Input: part model. Units: mm. Frame: model coordinates. A direction names the side the tool comes from. Give positions to 0.01 mm unless a question says otherwise; leave off trailing zeros. Loops run counter-clockwise (first coordinate to the right, second up) from the corner with the lowest first, then second, coordinate; pieces in that order, holes last. Notation, with made-up numbers: (5.5, 39.25) - (9.5, 39.25) arc R30 ccw to (9.5, 72.25) - close; hole circle Ø4 at (68, 68.25). An arc over 180 degrees is marked (long way). Answer as a JSON object with one key per item and string values.
from build123d import *

# Parameters (mm, degrees)
SKETCH3_W           = 29.5
SKETCH3_H           = 13
BOSS_EXTRUDE2_DEPTH = 7.2
SKETCH5_R           = 1.6
BOSS_EXTRUDE3_DEPTH = 1.5
SKETCH9_W           = 8.95
SKETCH9_H           = 11.9
SKETCH9_W_2         = 10.45
BOSS_EXTRUDE4_DEPTH = 14.4
SKETCH10_W          = 10.1
SKETCH10_H          = 8.4
BOSS_EXTRUDE5_DEPTH = 9.9
SKETCH11_W          = 6.95
SKETCH11_H          = 9.9
SKETCH11_W_2        = 8.45
CUT_EXTRUDE2_DEPTH  = 5
FILLET2_R           = 1


with BuildPart() as part:
    # Sketch3 → Boss-Extrude2 (new body)
    with BuildSketch(Plane(origin=(0, 0, 0), x_dir=(1, 0, 0), z_dir=(0, 1, 0))):
        Rectangle(SKETCH3_W, SKETCH3_H)
    extrude(amount=BOSS_EXTRUDE2_DEPTH)

    # Sketch5 → Boss-Extrude3 (add)
    with BuildSketch(Plane(origin=(0, 0, 0), x_dir=(1, 0, 0), z_dir=(0, 1, 0))):
        with BuildLine():
            Line((-18.5, 3.75), (-14.75, 3.75))
            Line((-14.75, 3.75), (-14.75, -3.75))
            Line((-14.75, -3.75), (-18.5, -3.75))
            ThreePointArc((-18.5, -3.75), (-22.25, 0), (-18.5, 3.75))
        make_face()
        with Locations(Location((-18.5, 0, 0), (0, 0, 270))):
            Circle(SKETCH5_R, mode=Mode.SUBTRACT)
    boss_extrude3 = extrude(amount=BOSS_EXTRUDE3_DEPTH)

    # Mirror1: Boss-Extrude3 across plane
    add(boss_extrude3.mirror(Plane(origin=(0, 0, 0), x_dir=(0, 0, 1), z_dir=(1, 0, 0))))

    # Sketch9 → Boss-Extrude4 (add)
    with BuildSketch(Plane(origin=(0, 7.2, 0), x_dir=(1, 0, 0), z_dir=(0, 1, 0))):
        with Locations((-10.275, 0)):
            Rectangle(SKETCH9_W, SKETCH9_H)
        with Locations((9.525, 0)):
            Rectangle(SKETCH9_W_2, SKETCH9_H)
    extrude(amount=BOSS_EXTRUDE4_DEPTH)

    # Sketch10 → Boss-Extrude5 (add)
    with BuildSketch(Plane(origin=(0, 7.2, 0), x_dir=(1, 0, 0), z_dir=(0, 1, 0))):
        with Locations((-0.75, -0.057461808)):
            Rectangle(SKETCH10_W, SKETCH10_H)
    extrude(amount=BOSS_EXTRUDE5_DEPTH)

    # Sketch11 → Cut-Extrude2 (cut)
    with BuildSketch(Plane(origin=(0, 21.6, 0), x_dir=(1, 0, 0), z_dir=(0, 1, 0))):
        with Locations((-10.275, 0)):
            Rectangle(SKETCH11_W, SKETCH11_H)
        with Locations((9.525, 0)):
            Rectangle(SKETCH11_W_2, SKETCH11_H)
    extrude(amount=-CUT_EXTRUDE2_DEPTH, mode=Mode.SUBTRACT)

    # Fillet2
    fillet2_edges = [part.edges().sort_by_distance(p)[0] for p in [
        (-14.75, 14.4, -5.95),
        (-14.75, 14.4, 5.95),
        (-5.8, 14.4, 5.95),
        (-5.8, 14.4, -5.95),
        (14.75, 14.4, 5.95),
        (14.75, 14.4, -5.95),
        (4.3, 14.4, -5.95),
        (4.3, 14.4, 5.95),
        (-13.75, 19.1, 4.95),
        (-13.75, 19.1, -4.95),
        (-6.8, 19.1, -4.95),
        (-6.8, 19.1, 4.95),
        (5.3, 19.1, 4.95),
        (5.3, 19.1, -4.95),
        (13.75, 19.1, -4.95),
        (13.75, 19.1, 4.95),
    ]]
    fillet(fillet2_edges, radius=FILLET2_R)


solid = part.part
Item 1: Cut plane A-A (z = 0). Return loops of the section in (x, y), then the cut area to 3 significant figures.
Geometry check:
{"outline": "(-22.25, 0) - (-20.1, 0) - (-20.1, 1.5) - (-22.25, 1.5) - close; (-16.9, 0) - (16.9, 0) - (16.9, 1.5) - (14.75, 1.5) - (14.75, 21.6) - (13.75, 21.6) - (13.75, 16.6) - (5.3, 16.6) - (5.3, 21.6) - (4.3, 21.6) - (4.3, 17.1) - (-5.8, 17.1) - (-5.8, 21.6) - (-6.8, 21.6) - (-6.8, 16.6) - (-13.75, 16.6) - (-13.75, 21.6) - (-14.75, 21.6) - (-14.75, 1.5) - (-16.9, 1.5) - close; (20.1, 0) - (22.25, 0) - (22.25, 1.5) - (20.1, 1.5) - close", "area": "528 mm2"}
Item 2: Material intervals for line 1 (X direction, y = 0.5, z = 0); line 2 (X direction, y = 17.25, z = -0.5); line 3 (X direction, y = 19.25, z = -4.25), sorted ascending. Write a range as [from, to].
Geometry check:
{"line 1": "x = [-22.25, -20.1], [-16.9, 16.9], [20.1, 22.25]", "line 2": "x = [-14.75, -13.75], [-6.8, -5.8], [4.3, 5.3], [13.75, 14.75]", "line 3": "x = [-14.75, -13.7], [-6.85, -5.8], [4.3, 5.35], [13.7, 14.75]"}
Item 3: Mould query, pull axis X, two halves, no side actions, for faces 5 (the face through (5.601, 19.065, -4.665)), 6 (the face through (17, 1, 3.75)). Classes: released by +X, released by -X, zero draft, split by the parting line, or undercut.
Geometry check:
{"face 5": "undercut", "face 6": "zero draft"}
Item 4: Contact query for flat-ended pins moving along their axis: P1, Ø1.5, axis at x = 8.5, y = 18, coming from the -Z side; P2, Ø2, axis at x = 10.5, y = 15.5, coming from the +Z side; P3, Ø3.5, axis at x = -9.5, z = 1.5, coming from the +Y side. Output: stop coordinate, or through.
Geometry check:
{"P1": "stops at z = -5.95", "P2": "stops at z = 5.95", "P3": "stops at y = 16.6"}
Item 5: Cut plane B-B (x = -1). Return loops of the section in (y, z), then the cut area to 3 significant figures.
Geometry check:
{"outline": "(0, -6.5) - (7.2, -6.5) - (7.2, -4.14) - (17.1, -4.14) - (17.1, 4.26) - (7.2, 4.26) - (7.2, 6.5) - (0, 6.5) - close", "area": "177 mm2"}
Item 6: Cut plane C-C (y = 9.5). Return loops of the section in (x, z).
Geometry check:
{"outline": "(-14.75, -4.95) arc R1 ccw to (-13.75, -5.95) - (-6.8, -5.95) arc R1 ccw to (-5.8, -4.95) - (-5.8, -4.14) - (4.3, -4.14) - (4.3, -4.95) arc R1 ccw to (5.3, -5.95) - (13.75, -5.95) arc R1 ccw to (14.75, -4.95) - (14.75, 4.95) arc R1 ccw to (13.75, 5.95) - (5.3, 5.95) arc R1 ccw to (4.3, 4.95) - (4.3, 4.26) - (-5.8, 4.26) - (-5.8, 4.95) arc R1 ccw to (-6.8, 5.95) - (-13.75, 5.95) arc R1 ccw to (-14.75, 4.95) - close"}
Item 7: Cut plane D-D (y = 3.25). Return loops of the section in (x, z), then the cut area to 4 significant figures.
Geometry check:
{"outline": "(-14.75, -6.5) - (14.75, -6.5) - (14.75, 6.5) - (-14.75, 6.5) - close", "area": "383.5 mm2"}
Item 8: Access query for faces 1 (the face through (9, 14, 5.95)), 2 (the face through (0, 7.2, -6)), 3 (the face through (-7.085, 19.065, -4.649)), 4 (the face through (0, 7.2, 6)). Directions: +Z, -Z, +X, -X, +Y, -Y. A direction counts if a zero-diameter tool reaches every point of the face in a straight line with its end or side. Return the directions, or none.
Geometry check:
{"face 1": "+Z, +X, -X, +Y", "face 2": "-Z, +Y", "face 3": "+Y", "face 4": "+Z, +Y"}
